The drawing under review shows one solid part. Ordinate dimensions are in mm from its lowest x, y, z. Coordinates: 2 decimals unless noted, no trailing zeros. Loops run counter-clockwise (first coordinate to the right, second up) from the corner with the lowest first, then second, coordinate; pieces in that order, holes last. Notation, with made-up numbers: (2, 40) - (42, 40) arc R24 cw to (42, 51) - close; hole circle Ø3 at (-32, 56.5). An arc over 180 degrees is marked (long way). Use one line per item in the form item = value. Start each with the question number.
1. To check wall thickness, follow probe 1 along Y at (x, z) = (22.5, 16.5); probe 2 along Y at (x, z) = (22, 60) (1 decimal); probe 3 along X at (y, z) = (22, 24) (1 decimal). State the ranges of each line that lie inside material, in increasing order.
2. Add section A-A on y = 22.5. Give the boundary of the cut face in (x, z).
3. Add section D-D on z = 22.5. Give the boundary of the cut face in (x, y), and give its area (3 significant figures).
4. For pin 1 Ø19 at (x, y) = (22.5, 22.5) entering from +Z; pin 2 Ø10 at (x, z) = (7, 49) entering from -Y; pin 3 Ø1 at (x, z) = (40, 22.5) entering from +Y; pin 4 Ø6 at (x, z) = (18.5, 25.5) entering from +Y, all flat-tipped, find the tip position at first contact; note any pin that passes through.
5. Add section C-C on z = 51. Give the boundary of the cut face in (x, y).
6. Draft analysis for pull direction Y (two halves, no side actions). For the marked faces 1, 2 and 3, state which applies: +Y half, -Y half, draft (parallel to the pull), parting line (faces both ways), or undercut.
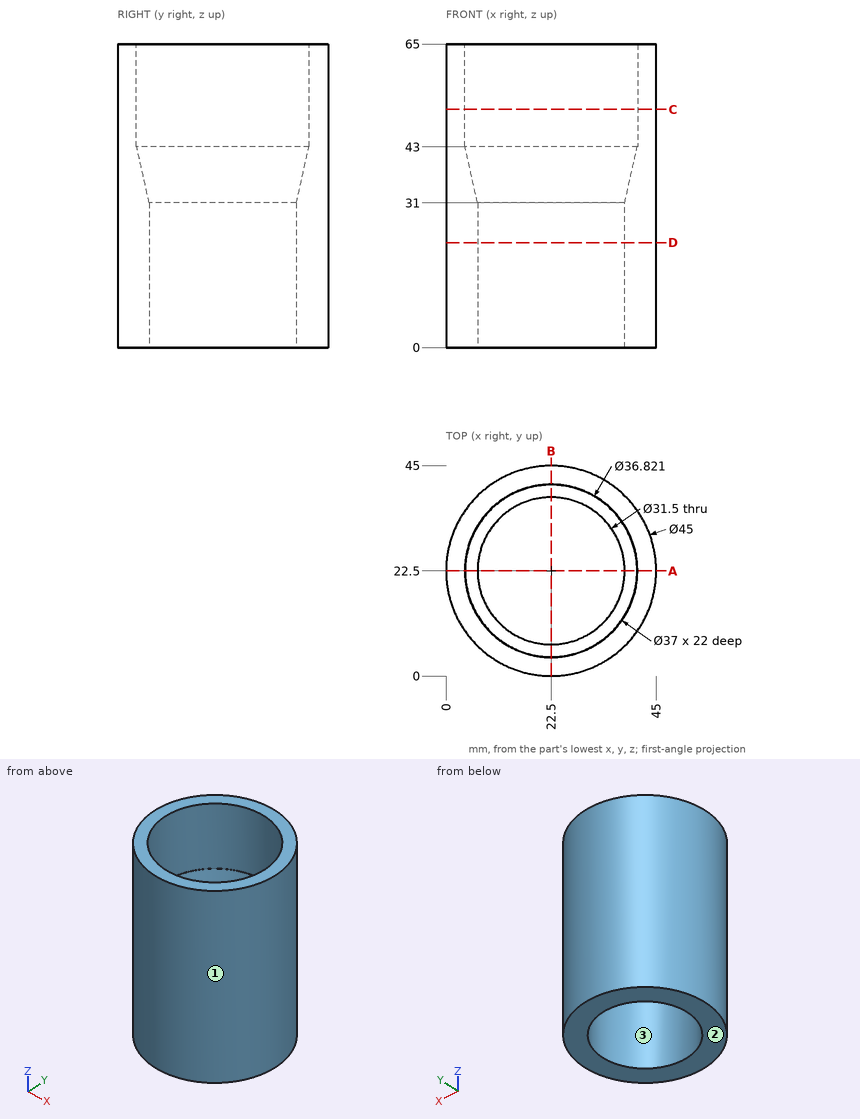
Conclusion:
q1.probe_1 = 0 to 6.75, 38.25 to 45
q1.probe_2 = 0 to 4, 41 to 45
q1.probe_3 = 0 to 6.8, 38.2 to 45
q2.outline = (0, 0) - (6.75, 0) - (6.75, 31) - (4.09, 43) - (4, 43) - (4, 65) - (0, 65) - close; (38.25, 0) - (45, 0) - (45, 65) - (41, 65) - (41, 43) - (40.91, 43) - (38.25, 31) - close
q3.outline = circle Ø45 at (22.5, 22.5); hole circle Ø31.5 at (22.5, 22.5)
q3.area = 811 mm^2
q4.pin_1 = through
q4.pin_2 = 2.6
q4.pin_3 = 37.24
q4.pin_4 = 44.98
q5.outline = circle Ø45 at (22.5, 22.5); hole circle Ø37 at (22.5, 22.5)
q6.face_1 = parting line
q6.face_2 = draft
q6.face_3 = undercut
